Work out the finished part from the listing and answer in its coordinate system (mm). Give positions to 0.01 mm unless a question says otherwise; leave off trailing zeros. Loops run counter-clockwise (first coordinate to the right, second up) from the corner with the lowest first, then second, coordinate; pieces in that order, holes last. Notation, with made-up numbers: (58.25, 70) - (73.25, 70) arc R25 cw to (73.25, 92) - close; hole circle Ø7 at (39.25, 19.5). An arc over 180 degrees is marked (long way). One line per item, written item: value.
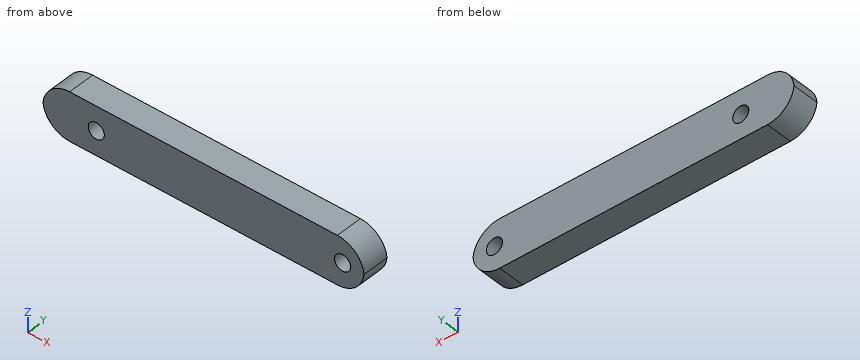
from build123d import *

# Parameters (mm, degrees)
F0_W        = 60
F0_H        = 9
F1_DEPTH    = 5
F2_T1_DEPTH = 30
F3_R        = 1.5
F4_DEPTH    = 12.5


# Not quite as in the source:
# - a fillet or chamfer that OpenCascade refuses, or shapes differently, is made with other operations: its cross-section is extruded or revolved along the edge and cut away or added


with BuildPart() as f1:
    # F0 (on Front) → F1 (new body)
    with BuildSketch(Plane.XZ):
        Rectangle(F0_W, F0_H)
    extrude(amount=F1_DEPTH)

    # F2: fillet of radius 5 on 4 edges, made by hand

    # F2_s2 → F2_t1 (cut)
    with BuildSketch(Plane.XZ.offset(-12.5)):
        with BuildLine():
            ThreePointArc((-25, 4.5), (-28.5355339059, 3.0355339059), (-30, -0.5))
            Line((-30, -0.5), (-30, 4.5))
            Line((-30, 4.5), (-25, 4.5))
        make_face()
        with BuildLine():
            ThreePointArc((-30, 0.5), (-28.5355339059, -3.0355339059), (-25, -4.5))
            Line((-25, -4.5), (-30, -4.5))
            Line((-30, -4.5), (-30, 0.5))
        make_face()
        with BuildLine():
            ThreePointArc((25, 4.5), (28.5355339059, 3.0355339059), (30, -0.5))
            Line((30, -0.5), (30, 4.5))
            Line((30, 4.5), (25, 4.5))
        make_face()
        with BuildLine():
            ThreePointArc((25, -4.5), (28.5355339059, -3.0355339059), (30, 0.5))
            Line((30, 0.5), (30, -4.5))
            Line((30, -4.5), (25, -4.5))
        make_face()
    extrude(amount=F2_T1_DEPTH, mode=Mode.SUBTRACT)

    # F3 (on Front) → F4 (cut, symmetric)
    with BuildSketch(Plane.XZ):
        with Locations((25.9749371855, 0)):
            Circle(F3_R)
        with Locations((-20.0250628145, 0)):
            Circle(F3_R)
    extrude(amount=F4_DEPTH, both=True, mode=Mode.SUBTRACT)


solid = f1.part
1. Section B-B (z = -1) is taken. Write down the section's boundary in (x, y), and give its area (3 significant figures).
Output:
outline: (-29.77, -5) - (-21.14, -5) - (-21.14, 0) - (-29.77, 0) - close; (-18.91, -5) - (24.86, -5) - (24.86, 0) - (-18.91, 0) - close; (27.09, -5) - (29.77, -5) - (29.77, 0) - (27.09, 0) - close
area: 275 mm²
2. A flat-ended cylindrical pin translates along its axis: pin 1 Ø4 at (x, z) = (25.97, 0) entering from -Y. Find the tip coordinate at first contact, or state that the pin passes through.
Output:
pin 1: stops at y = -5
3. Section A-A (y = -1.65) is taken. Write down the section's boundary in (x, z), and give its area (3 significant figures).
Output:
outline: (-29.97, 0) arc R5 ccw to (-25, -4.5) - (25, -4.5) arc R5 ccw to (29.97, 0) arc R5 ccw to (25, 4.5) - (-25, 4.5) arc R5 ccw to start; hole circle Ø3 at (-20.03, 0); hole circle Ø3 at (25.97, 0)
area: 504 mm²
4. Find the intervals of material crossed by line 1 along X through (y, z) = (-4.3, -1); line 2 along X through (y, z) = (-1.05, -1.25); line 3 along Z through (x, y) = (26.5, -4.7), in increasing order.
Output:
line 1: x = -29.77 to -21.14, -18.91 to 24.86, 27.09 to 29.77
line 2: x = -29.68 to -20.85, -19.2 to 25.15, 26.8 to 29.68
line 3: z = -4.27 to -1.41, 1.41 to 4.27
